from build123d import *

# Parameters (mm, degrees)
SKETCH_1_W          = 5
SKETCH_1_H          = 7
EXTRUDE_2_DEPTH     = 140
FILLET_1_R          = 3.5
SKETCH_3_R          = 1.55
CUT_EXTRUDE_1_DEPTH = 141.132972565
SKETCH_4_W          = 2.5
SKETCH_4_H          = 7
EXTRUDE_3_DEPTH     = 7
SKETCH_5_W          = 15
SKETCH_5_H          = 7
EXTRUDE_4_DEPTH     = 1
FILLET_2_R          = 3.5
SKETCH_6_R          = 1.5
CUT_EXTRUDE_2_DEPTH = 148.083309726
FILLET_3_R          = 3.5


# Some blends are built 0.0001 mm under size
with BuildPart() as part:
    # 草图1 → 凸台-拉伸2 (new body)
    with BuildSketch(Plane.XY):
        Rectangle(SKETCH_1_W, SKETCH_1_H)
    extrude(amount=EXTRUDE_2_DEPTH)

    # 圆角1
    fillet_1_edges = [part.edges().sort_by_distance(p)[0] for p in [
        (0, -3.5, 0),
        (0, 3.5, 0),
    ]]
    fillet(fillet_1_edges, radius=FILLET_1_R - 0.0001)  # a hair under: the kernel refuses the full size

    # 草图3 → 切除-拉伸1 (cut, through all)
    with BuildSketch(Plane(origin=(2.5, 0, 0), x_dir=(0, 0, -1), z_dir=(1, 0, 0))):
        with Locations(Location((-3.5, 0, 0), (0, 0, 90))):
            Circle(SKETCH_3_R)
    extrude(amount=-CUT_EXTRUDE_1_DEPTH, mode=Mode.SUBTRACT)

    # 草图4 → 凸台-拉伸3 (add)
    with BuildSketch(Plane.XY.offset(140)):
        with Locations((1.25, 0)):
            Rectangle(SKETCH_4_W, SKETCH_4_H)
    extrude(amount=EXTRUDE_3_DEPTH)

    # 草图5 → 凸台-拉伸4 (add)
    with BuildSketch(Plane(origin=(2.5, 0, 0), x_dir=(0, 0, -1), z_dir=(1, 0, 0))):
        with Locations((-139.5, 0)):
            Rectangle(SKETCH_5_W, SKETCH_5_H)
    extrude(amount=EXTRUDE_4_DEPTH)

    # 圆角2
    fillet_2_edges = [part.edges().sort_by_distance(p)[0] for p in [
        (1.75, -3.5, 147),
        (1.75, 3.5, 147),
    ]]
    fillet(fillet_2_edges, radius=FILLET_2_R - 0.0001)  # a hair under: the kernel refuses the full size

    # 草图6 → 切除-拉伸2 (cut, through all)
    with BuildSketch(Plane.ZY):
        with Locations(Location((143.5, 0, 0), (0, 0, 270))):
            Circle(SKETCH_6_R)
    extrude(amount=-CUT_EXTRUDE_2_DEPTH, mode=Mode.SUBTRACT)

    # 圆角3
    # the kernel refuses this fillet: 3.5 mm, written as the material it adds along each edge
    with BuildSketch(Plane(origin=(2.5, 3.5, 132), x_dir=(1, 0, 0), z_dir=(0, -1, 0))) as fillet_3_piece_1:
        with BuildLine():
            CenterArc((3.5, -2.449489743), FILLET_3_R, 135.584691403, 44.415308597)
            Line((0, -2.449489743), (-0.07, -2.449489743))
            Line((-0.07, -2.449489743), (-0.07, 0))
            Line((-0.07, 0), (0, 0.07))
            ThreePointArc((0, 0.07), (0.5, 0.07), (0.95, 0.048989795))
            Line((0.95, 0.048989795), (1, 0))
        make_face()
    extrude(amount=7)


solid = part.part
Verification items for the finished model (mm, model axes). A direction names the side the tool comes from. Give positions to 0.01 mm unless a question says otherwise; leave off trailing zeros. Loops run counter-clockwise (first coordinate to the right, second up) from the corner with the lowest first, then second, coordinate; pieces in that order, holes last. Notation, with made-up numbers: (83.25, 28) - (94.25, 28) arc R33 ccw to (94.25, 58) - close; hole circle Ø4 at (-14.75, 85). An arc over 180 degrees is marked (long way). Write item = value, one per line. Start each with the question number.
Q1. Cross-section at A-A, the plane x = 1.1. State how many separate pieces and enclosed holes the cut face has, and give its area (3 significant figures).
Q2. Mould release check, pull along Y, two halves, no side actions. Record for faces 4 (the face through (-2.5, 0, 69)), 5 (the face through (0, -3.5, 74)), 6 (the face through (2, 0, 145)): released by +Y, released by -Y, zero draft, split by the parting line, or undercut.
Q3. Thickness scan on line 1 (Z direction, x = 0.75, y = 0); line 2 (Y direction, x = 1.4, z = 143.5); line 3 (Z direction, x = -0.25, y = 0). Record the ranges inside material, lowest first.
Q4. Tool access check on faces 1 (the face through (2.5, 0, 64)), 2 (the face through (0.04, -2.5, 1.05)), 3 (the face through (-1, 0, 140)). Record the directions out of +Z, -Z, +X, -X, +Y, -Y that give a thin tool (end or side, any length) a straight path to the whole face; none if there is none.
Q5. Cross-section at B-B, the plane z = 113.5. Enter the section's corners in (x, y).
Q6. Depth check by flat-ended pin: P1, Ø3, axis at x = -1.5, y = 2, coming from the -Z side; P2, Ø2, axis at y = 0, z = 114.5, coming from the +X side; P3, Ø2.5, axis at y = 0, z = 3.5, coming from the -X side; P4, Ø1.2, axis at x = -0.5, y = 1, coming from the +Z side. Enter the tip coordinate at first touch or a pass-through.
Answer key:
q1.separate_pieces = 1
q1.enclosed_holes = 2
q1.area = 1,000 mm^2
q2.face_4 = zero draft
q2.face_5 = released by -Y
q2.face_6 = undercut
q3.line_1 = 0 to 1.95, 5.05 to 142, 145 to 147
q3.line_2 = -3.5 to -1.5, 1.5 to 3.5
q3.line_3 = 0 to 1.95, 5.05 to 140
q4.face_1 = -Z, +X, +Y, -Y
q4.face_2 = -Z, +X, -X, -Y
q4.face_3 = +Z, -X, +Y, -Y
q5.outline = (-2.5, -3.5) - (2.5, -3.5) - (2.5, 3.5) - (-2.5, 3.5) - close
q6.P1 = 0.04
q6.P2 = 2.5
q6.P3 = through
q6.P4 = 146.94
